from build123d import *

# Parameters (mm, degrees)
F0_W     = 30
F0_H     = 30
F0_R     = 2.5
F1_DEPTH = 12.5
F2_R     = 2
F3_W     = 10.5
F3_H     = 6
F3_W_2   = 6
F3_H_2   = 10.5
F4_DEPTH = 25
F5_DEPTH = 25
F7_DEPTH = 25
F8_R     = 2
F9_R     = 0.7
F10_R    = 5


with BuildPart() as f1:
    # F0 (on Front) → F1 (new body, symmetric)
    with BuildSketch(Plane.XZ):
        Rectangle(F0_W, F0_H)
        Circle(F0_R, mode=Mode.SUBTRACT)
    extrude(amount=F1_DEPTH, both=True)

    # F2
    f2_edges = [f1.edges().sort_by_distance(p)[0] for p in [
        (15, 0, 15),
        (-15, 0, 15),
        (-15, 0, -15),
        (15, 0, -15),
    ]]
    fillet(f2_edges, radius=F2_R)

    # F3 (on face) → F4 (cut)
    with BuildSketch(Plane.XZ.offset(12.5)):
        with Locations((9.75, 0)):
            Rectangle(F3_W, F3_H)
        with Locations((0, 9.75)):
            Rectangle(F3_W_2, F3_H_2)
        with Locations((0, -9.75)):
            Rectangle(F3_W_2, F3_H_2)
        with Locations((-9.75, 0)):
            Rectangle(F3_W, F3_H)
    extrude(amount=-F4_DEPTH, mode=Mode.SUBTRACT)

    # F3 (on face) → F5 (cut)
    with BuildSketch(Plane.XZ.offset(12.5)):
        with Locations((9.75, 0)):
            Rectangle(F3_W, F3_H)
        with Locations((0, 9.75)):
            Rectangle(F3_W_2, F3_H_2)
        with Locations((0, -9.75)):
            Rectangle(F3_W_2, F3_H_2)
        with Locations((-9.75, 0)):
            Rectangle(F3_W, F3_H)
    extrude(amount=-F5_DEPTH, mode=Mode.SUBTRACT)

    # F6 (on face) → F7 (cut)
    with BuildSketch(Plane.XZ.offset(12.5)):
        Polygon((3, 13.5), (3, 4.5), (12, 13.5), align=None)
        Polygon((13.5, 12), (4.5, 3), (13.5, 3), align=None)
        Polygon((3, -4.5), (3, -13.5), (12, -13.5), align=None)
        Polygon((13.5, -3), (4.5, -3), (13.5, -12), align=None)
        Polygon((-3, 4.5), (-3, 13.5), (-12, 13.5), align=None)
        Polygon((-13.5, 3), (-4.5, 3), (-13.5, 12), align=None)
        Polygon((-13.5, -12), (-4.5, -3), (-13.5, -3), align=None)
        Polygon((-3, -13.5), (-3, -4.5), (-12, -13.5), align=None)
    extrude(amount=-F7_DEPTH, mode=Mode.SUBTRACT)

    # F8
    f8_edges = [f1.edges().sort_by_distance(p)[0] for p in [
        (-12, 0, -13.5),
        (12, 0, -13.5),
        (13.5, 0, -12),
        (-13.5, 0, -12),
        (13.5, 0, 12),
        (12, 0, 13.5),
        (-13.5, 0, 12),
        (-12, 0, 13.5),
    ]]
    fillet(f8_edges, radius=F8_R)

    # F9
    f9_edges = [f1.edges().sort_by_distance(p)[0] for p in [
        (13.5, 0, 3),
        (15, 0, 3),
        (15, 0, -3),
        (13.5, 0, -3),
        (3, 0, -15),
        (-3, 0, -15),
        (3, 0, -13.5),
        (-3, 0, -13.5),
        (-15, 0, -3),
        (-13.5, 0, -3),
        (-15, 0, 3),
        (-13.5, 0, 3),
        (3, 0, 13.5),
        (3, 0, 15),
        (-3, 0, 15),
        (-3, 0, 13.5),
    ]]
    fillet(f9_edges, radius=F9_R)

    # F10
    f10_edges = [f1.edges().sort_by_distance(p)[0] for p in [
        (4.5, 0, -3),
        (4.5, 0, 3),
        (-3, 0, -4.5),
        (3, 0, -4.5),
        (-4.5, 0, -3),
        (-4.5, 0, 3),
        (3, 0, 4.5),
        (-3, 0, 4.5),
    ]]
    fillet(f10_edges, radius=F10_R)


solid = f1.part
Work out the finished part from the listing and answer in its coordinate system (mm). A direction names the side the tool comes from. Round coordinates to 2 decimals unless told otherwise and drop trailing zeros. Loops run counter-clockwise (first coordinate to the right, second up) from the corner with the lowest first, then second, coordinate; pieces in that order, holes last. Notation, with made-up numbers: M -18,34.25 L 35,34.25 A22 ccw 35,73.25 Z; hole C 27.25,77 d3. An arc over 180 degrees is marked long. One line per question, with ' | ' between items. Start each with the question number.
(1) Flat-ended cylindrical pins translate along their axes: pin 1 Ø0.6 at (x, y) = (-0.5, 4.5) entering from +Z; pin 2 Ø2 at (y, z) = (-4, 0) entering from -X. Find the tip coordinate at first contact, or state that the pin passes through.
(2) A cutting plane is placed at A-A on z = 0. Write down the section's boundary in (x, y).
(3) For a pull along Z with two mould halves and no side action, classify faces 4 (the face through (15, 0, 8)), 5 (the face through (-6.5, -0.2, -8)), 6 (the face through (14.43, 0.18, 14.4)), 7 (the face through (13.5, 0, -5)) as released by +Z, released by -Z, zero draft, split by the parting line, or undercut.
(4) A tool of negligible diameter and unlimited length cuts with its end or side. For faces 1 (the face through (-2.87, 0.18, 4.89)), 2 (the face through (-15, 0, -8)), 3 (the face through (-4.5, 0, 0)), from which of +Z, -Z, +X, -X, +Y, -Y can it reach the whole face along a straight path? Write none if from no direction.
(5) Find the intervals of material crossed by line 1 (X direction, y = 5.25, z = -11.5); line 2 (Z direction, x = 0, y = -1); line 3 (Z direction, x = -6.25, y = -5.25), in increasing order.
(6) A cutting plane is placed at B-B on x = 0. Write down the section's boundary in (y, z), plus the area to 3 significant figures.
Geometry check:
1) pin 1: stops at z = 4.5 | pin 2: stops at x = -4.5
2) outline: M -4.5,-12.5 L -2.5,-12.5 L -2.5,12.5 L -4.5,12.5 Z; M 2.5,-12.5 L 4.5,-12.5 L 4.5,12.5 L 2.5,12.5 Z
3) face 4: zero draft | face 5: undercut | face 6: released by +Z | face 7: undercut
4) face 1: +Y, -Y | face 2: +Z, -Z, -X, +Y, -Y | face 3: -X, +Y, -Y
5) line 1: x = -15 to -9.17, 9.17 to 15 | line 2: z = -4.5 to -2.5, 2.5 to 4.5 | line 3: z = -15 to -13.5, -7.75 to -4.75, 4.75 to 7.75, 13.5 to 15
6) outline: M -12.5,-4.5 L 12.5,-4.5 L 12.5,-2.5 L -12.5,-2.5 Z; M -12.5,2.5 L 12.5,2.5 L 12.5,4.5 L -12.5,4.5 Z | area: 100 mm²
